Autodesk Inventor part; units mm, degrees
ref_plane "MSC_PF1" through (0, 0, 0) normal (1, 0, 0) x (0, 1, 0)
ref_plane "MSC_PT1" through (0, 0, 0) normal (0, 0, -1) x (-1, 0, 0)
ref_plane "YZ Plane" through (0, 0, 0) normal (1, 0, 0) x (0, 1, 0)
sketch "Sketch2" plane through (0, 0, 0) normal (0, 0, 1) x (1, 0, 0)
  circle A0 centre (0, 0) radius 1.65
  dimension "d3" = 3.3
extrude "Extrusion1" add sketch "Sketch2" against normal blind 1.31
sketch "Sketch3" plane through (0, 0, -1.31) normal (0, 0, -1) x (-1, 0, 0)
  circle A0 centre (0, 0) radius 2
  circle A1 centre (0, 0) radius 1.65 construction
  dimension "d28" = 360
  dimension "d9" = 4
extrude "Extrusion2" add sketch "Sketch3" along normal blind 10.69
chamfer "Chamfer1" distance 0.35 distance2 0.35 1 edges at (2, 0, -1.31) measured on face at (-1.848, -0.2912, -1.31)
sketch "Sketch4" plane through (0, 0, 0) normal (0, 0, 1) x (1, 0, 0)
  circle A0 centre (0, 0) radius 4.15
  circle A1 centre (0, 0) radius 1.65 construction
  dimension "d15" = 8.3
extrude "Extrusion3" add sketch "Sketch4" along normal blind 1.7
fillet "Fillet1" radius 0.2 1 edges at (-1.65, 0, 0)
sketch "Sketch5" plane through (0, 0, 0) normal (0, 1, 0) x (-1, 0, 0)
  line L0 (4.15, 1.7) -> (4.15, 0)
  line L1 (4.0013, 1.7) -> (4.15, 1.7)
  line L2 (4.15, 0) -> (4.0013, 1.7)
  line L3 (-4.15, 1.7) -> (4.15, 1.7) construction
  line L4 (-4.15, 0) -> (4.15, 0) construction
  line L5 (0, -0.34) -> (0, 2.04)
  line L6 (5.81, 0) -> (-5.81, 0)
  dimension "d20" = 5
  dimension "d56" = 4.15
  dimension "d57" = 1.7
revolve "Revolution1" cut sketch "Sketch5" angle 360 about axis through (0, 0, -10) along (0, 0, 1)
sketch "Sketch6" plane through (0, 0, 0) normal (0, 1, 0) x (-1, 0, 0)
  line L0 (0, 2.5) -> (0, 1.7)
  arc A0 (4.0013, 1.7) -> (0, 2.5) centre (-1.2292, -14.0544) ccw
  line L1 (0, 1.7) -> (4.0013, 1.7)
  line L2 (4.0013, 1.7) -> (-4.0013, 1.7) construction
  line L3 (0, -4.4495) -> (0, 0.4495)
  line L4 (0, -17.39) -> (0, 5.959)
  line L5 (5.6314, 0) -> (-5.6067, 0)
  dimension "d58" = 0.8
  dimension "d59" = 4.0013
  dimension "d60" = 0
  dimension "d62" = 16.6
revolve "Revolution2" add sketch "Sketch6" angle 360 about axis through (0, 0, -4.4495) along (0, 0, 1)
sketch "Sketch7" plane through (0, 0, 0) normal (0, 1, 0) x (-1, 0, 0)
  line L0 (2.15, 2.5) -> (-2.15, 2.5)
  line L1 (1.1568, 0.37) -> (2.15, 2.5)
  line L2 (-1.1568, 0.37) -> (1.1568, 0.37)
  line L3 (-2.15, 2.5) -> (-1.1568, 0.37)
  line L4 (0, -0.056) -> (0, 2.926)
  line L5 (3.01, 0) -> (-3.01, 0)
  dimension "d32" = 2.13
  dimension "d34" = 65
  dimension "d36" = 65
  dimension "d63" = 2.15
  dimension "d64" = 2.5
  dimension "d65" = 4.3
extrude "Extrusion4" cut sketch "Sketch7" against normal mid plane 1.4333
sketch "Sketch8" plane through (0, 0, 0) normal (1, 0, 0) x (0, 1, 0)
  line L0 (-1.1568, 0.37) -> (-2.15, 2.5)
  line L1 (1.1568, 0.37) -> (-1.1568, 0.37)
  line L2 (2.15, 2.5) -> (1.1568, 0.37)
  line L3 (-2.15, 2.5) -> (2.15, 2.5)
  line L4 (0, -0.056) -> (0, 2.926)
  line L5 (-3.01, 0) -> (3.01, 0)
  dimension "d40" = 65
  dimension "d42" = 65
  dimension "d44" = 2.13
  dimension "d66" = 4.3
  dimension "d67" = 2.5
  dimension "d69" = 2.15
extrude "Extrusion5" cut sketch "Sketch8" along normal mid plane 1.4333
sketch "Sketch9" plane through (0, 0, 0) normal (0, 1, 0) x (-1, 0, 0)
  line L0 (0, 2.5) -> (0, 0.37)
  line L1 (1.72, 2.5) -> (0, 2.5)
  line L2 (0, 0.37) -> (1.72, 2.5)
  line L3 (-4.15, 0) -> (4.15, 0) construction
  line L4 (0, -0.5) -> (0, 3)
  line L5 (5.81, 0) -> (-5.81, 0)
  dimension "d50" = 2.13
  dimension "d52" = 2.13
  dimension "d54" = 1.72
  dimension "d70" = 0
  dimension "d71" = 2.5
revolve "Revolution3" cut sketch "Sketch9" angle 360 about axis through (0, 0, -10) along (0, 0, 1)
thread "Thread1"
ref_plane "MSC_PF1" through (0, 0, 0) normal (1, 0, 0) x (0, 1, 0)
ref_plane "MSC_PT1" through (0, 0, 0) normal (0, 0, -1) x (-1, 0, 0)
equation "\"d12\" = -0.5 * msp_ds + 0.5 * NND"
equation "\"d13\" = 0.5 * NND - 0.5 * msp_ds"
equation "\"d18\" = r"
equation "\"d4\" = -b + NLG"
equation "\"d9\" = NND"
equation "\"d10\" = b"
equation "\"d15\" = Dk"
equation "\"d16\" = ParK"
equation "\"d32\" = q"
equation "\"d63\" = 0.5 * M"
equation "\"d64\" = ParK + ParF"
equation "\"d65\" = M"
equation "\"d37\" = 2 * msp_s"
equation "\"d44\" = q"
equation "\"d66\" = M"
equation "\"d67\" = ParK + ParF"
equation "\"d69\" = 0.5 * M"
equation "\"d47\" = 2 * msp_s"
equation "\"d3\" = msp_ds"
equation "\"d56\" = 0.5 * Dk"
equation "\"d57\" = ParK"
equation "\"d58\" = ParF"
equation "\"d59\" = 0.5 * Dk - msp_v"
equation "\"d62\" = 2 * Dk"
equation "\"d50\" = q"
equation "\"d52\" = q"
equation "\"d54\" = msp_rr"
equation "\"d71\" = ParK + ParF"
equation "\"PTC\" = 0.7"
equation "\"NLG\" = 12"
equation "\"Dk\" = 8.3"
equation "\"ParK\" = 1.7"
equation "\"NND\" = 4"
equation "\"M\" = 4.3"
equation "\"q\" = 2.13"
equation "\"r\" = 0.2"
equation "\"msp_ds\" = NND - PTC"
equation "\"b\" = 10.69"
equation "\"msp_x\" = 1.25 * PTC"
equation "\"msp_s\" = 0.166667 * M"
equation "\"msp_rr\" = 0.4 * M"
equation "\"ParF\" = 0.8"
equation "\"msp_v\" = 0.0874887 * ParK"
equation "\"THREADDIA\" = NND"
properties part number "JIS B 1111 - M4x12" material "Steel, Mild"
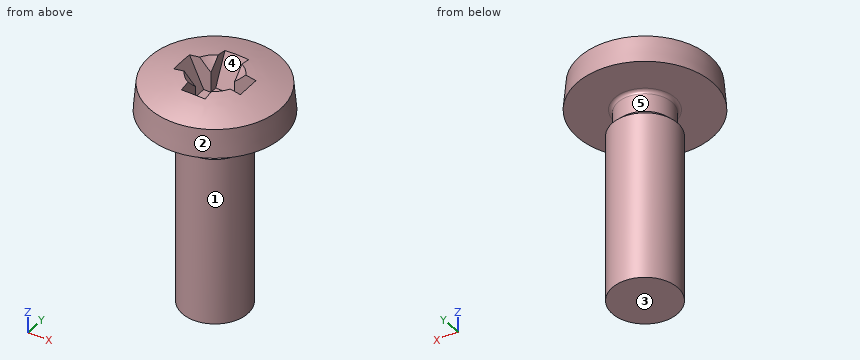
Verification items for the finished model (mm, model axes). Face numbers are marked on the shaded views. A direction names the side the tool comes from. Give positions to 0.01 mm unless a question says otherwise; leave off trailing zeros. Write each loop counter-clockwise with the first axis right and the second up, starting at its lowest first coordinate (ties: lowest second). Pieces come first, ordered by that corner, then holes. Notation, with made-up numbers: M 26,-20.5 L 39,-20.5 A21 cw 39,6.5 Z; hole C -2,77 d5. An arc over 180 degrees is marked long. Put each result on its own line as item: value. Start each with the question number.
1. Section check A-A (z = -5.75). Record the cut outline in (x, y).
2. Go/stop test with flat-tipped pins: pin 1 Ø1.5 at (x, z) = (-3, -3.5) entering from +Y (1 decimal); pin 2 Ø1.9 at (x, y) = (0.5, 0) entering from +Z; pin 3 Ø0.6 at (x, z) = (-1.5, 1) entering from -Y; pin 4 Ø3 at (y, z) = (-2.5, 0) entering from -X. Record where each tip stops, or that it passes through.
3. Set-up check for the marked faces 1 and 2: record each of +Z, -Z, +X, -X, +Y, -Y from which the full face is reachable in a straight line by a thin tool's end or side.
4. Scan lines: line 1 along Z through (x, y) = (-0.25, 0); line 2 along Z through (x, y) = (-2, -0.75); line 3 along X through (y, z) = (-0.25, -9.75). Record each from-to range of solid material in increasing order. Write a range as [from, to].
5. Draft check along Y on the marked faces 3, 4 and 5. Enter one of: +Y half, -Y half, draft (parallel to the pull), parting line (faces both ways), or undercut.
Answer list:
1. outline: C 0,0 d4
2. pin 1: through
2. pin 2: z = 2.02
2. pin 3: y = -3.89
2. pin 4: x = -4.03
3. face 1: -Z
3. face 2: +Z
4. line 1: [-12, 0.37]
4. line 2: [0, 2.2]
4. line 3: [-1.98, 1.98]
5. face 3: draft
5. face 4: undercut
5. face 5: parting line
